CAD build for the part. Positions are in the model's coordinates, mm. A direction names the side the tool comes from. Coordinates: 2 decimals unless noted, no trailing zeros. Order: outer loops, then holes, each group sorted by start corner. A loop starts at its lowest first (then second) coordinate and runs counter-clockwise, first axis right, second up. Notation, with made-up numbers: M -11.5,32.25 L 25.5,32.25 A16 ccw 25.5,44.25 Z; hole C 26,76.25 d3. An arc over 180 degrees is marked long. One line per item, written item: value.
from build123d import *

# Parameters (mm, degrees)
SKETCH1_W           = 244
SKETCH1_H           = 158.154567899
BOSS_EXTRUDE2_DEPTH = 5
SKETCH2_W           = 28.286613298
SKETCH2_H           = 62.131328865
CUT_EXTRUDE1_DEPTH  = 10
SKETCH7_W           = 32
SKETCH7_H           = 84.5
CUT_EXTRUDE5_DEPTH  = 10
SKETCH9_R           = 1.5
CUT_EXTRUDE7_DEPTH  = 10
SKETCH10_W          = 26
SKETCH10_H          = 40
CUT_EXTRUDE8_DEPTH  = 10
SKETCH12_W          = 92
SKETCH12_H          = 45
CUT_EXTRUDE10_DEPTH = 10
SKETCH13_R          = 2.5
CUT_EXTRUDE11_DEPTH = 10
CUT_EXTRUDE12_DEPTH = 10
SKETCH15_W          = 32
SKETCH15_H          = 26
BOSS_EXTRUDE3_DEPTH = 5
SKETCH16_R          = 1.5
CUT_EXTRUDE13_DEPTH = 10
SKETCH17_R          = 1.5
CUT_EXTRUDE14_DEPTH = 10
SKETCH19_R          = 2
CUT_EXTRUDE16_DEPTH = 10
SKETCH20_W          = 22
SKETCH20_H          = 28
CUT_EXTRUDE17_DEPTH = 10
CUT_EXTRUDE18_DEPTH = 10


with BuildPart() as part:
    # Sketch1 → Boss-Extrude2 (new body)
    with BuildSketch(Plane.XY):
        with Locations((-3, -45.239754423)):
            Rectangle(SKETCH1_W, SKETCH1_H)
    extrude(amount=BOSS_EXTRUDE2_DEPTH)

    # Sketch2 → Cut-Extrude1 (cut)
    with BuildSketch(Plane(origin=(0, 0, 0), x_dir=(-1, 0, 0), z_dir=(0, 0, -1))):
        with Locations((50, -93.25137394)):
            Rectangle(SKETCH2_W, SKETCH2_H)
    extrude(amount=-CUT_EXTRUDE1_DEPTH, mode=Mode.SUBTRACT)

    # Sketch7 → Cut-Extrude5 (cut)
    with BuildSketch(Plane(origin=(0, 0, 0), x_dir=(-1, 0, 0), z_dir=(0, 0, -1))):
        with Locations((-103, -40.912470473)):
            Rectangle(SKETCH7_W, SKETCH7_H)
    extrude(amount=-CUT_EXTRUDE5_DEPTH, mode=Mode.SUBTRACT)

    # Sketch9 → Cut-Extrude7 (cut)
    with BuildSketch(Plane(origin=(0, 0, 0), x_dir=(-1, 0, 0), z_dir=(0, 0, -1))):
        with Locations((31.026566737, -67.835709507)):
            Circle(SKETCH9_R)
        with Locations((31.026566737, -82.835709507)):
            Circle(SKETCH9_R)
    extrude(amount=-CUT_EXTRUDE7_DEPTH, mode=Mode.SUBTRACT)

    # Sketch10 → Cut-Extrude8 (cut)
    with BuildSketch(Plane(origin=(0, 0, 0), x_dir=(-1, 0, 0), z_dir=(0, 0, -1))):
        with Locations((3, -104.317038372)):
            Rectangle(SKETCH10_W, SKETCH10_H)
    extrude(amount=-CUT_EXTRUDE8_DEPTH, mode=Mode.SUBTRACT)

    # Sketch12 → Cut-Extrude10 (cut)
    with BuildSketch(Plane(origin=(0, 0, 0), x_dir=(-1, 0, 0), z_dir=(0, 0, -1))):
        with Locations((-3, 11.337529527)):
            Rectangle(SKETCH12_W, SKETCH12_H)
    extrude(amount=-CUT_EXTRUDE10_DEPTH, mode=Mode.SUBTRACT)

    # Sketch13 → Cut-Extrude11 (cut)
    with BuildSketch(Plane(origin=(0, 0, 0), x_dir=(-1, 0, 0), z_dir=(0, 0, -1))):
        with Locations((-107, -109.317038372)):
            Circle(SKETCH13_R)
        with Locations((113, -109.317038372)):
            Circle(SKETCH13_R)
        with Locations((-62, 13.837529527)):
            Circle(SKETCH13_R)
        with Locations((68, 13.837529527)):
            Circle(SKETCH13_R)
    extrude(amount=-CUT_EXTRUDE11_DEPTH, mode=Mode.SUBTRACT)

    # Sketch14 → Cut-Extrude12 (cut)
    with BuildSketch(Plane(origin=(0, 0, 0), x_dir=(-1, 0, 0), z_dir=(0, 0, -1))):
        Polygon((-119, -94.885674772), (-119, -98.885674772), (-111.613125162, -98.885674772), (-111.613125162, -99.635674772), (-109.213125162, -99.635674772), (-109.213125162, -98.885674772), (-102, -98.885674772), (-102, -94.885674772), (-109.213125162, -94.885674772), (-109.213125162, -94.135674772), (-111.613125162, -94.135674772), (-111.613125162, -94.885674772), align=None)
        Polygon((-102, 11.114325228), (-109.213125162, 11.114325228), (-109.213125162, 11.864325228), (-111.613125162, 11.864325228), (-111.613125162, 11.114325228), (-119, 11.114325228), (-119, 7.114325228), (-111.613125162, 7.114325228), (-111.613125162, 6.364325228), (-109.213125162, 6.364325228), (-109.213125162, 7.114325228), (-102, 7.114325228), align=None)
        Polygon((117.613125162, 7.114325228), (125, 7.114325228), (125, 11.114325228), (117.613125162, 11.114325228), (117.613125162, 11.864325228), (115.213125162, 11.864325228), (115.213125162, 11.114325228), (108, 11.114325228), (108, 7.114325228), (115.213125162, 7.114325228), (115.213125162, 6.364325228), (117.613125162, 6.364325228), align=None)
        Polygon((117.613125162, -98.885674772), (125, -98.885674772), (125, -94.885674772), (117.613125162, -94.885674772), (117.613125162, -94.135674772), (115.213125162, -94.135674772), (115.213125162, -94.885674772), (108, -94.885674772), (108, -98.885674772), (115.213125162, -98.885674772), (115.213125162, -99.635674772), (117.613125162, -99.635674772), align=None)
    extrude(amount=-CUT_EXTRUDE12_DEPTH, mode=Mode.SUBTRACT)

    # Sketch15 → Boss-Extrude3 (add)
    with BuildSketch(Plane(origin=(0, 0, 0), x_dir=(-1, 0, 0), z_dir=(0, 0, -1))):
        with Locations((-103, -11.662470473)):
            Rectangle(SKETCH15_W, SKETCH15_H)
    extrude(amount=-BOSS_EXTRUDE3_DEPTH)

    # Sketch16 → Cut-Extrude13 (cut)
    with BuildSketch(Plane(origin=(0, 0, 0), x_dir=(-1, 0, 0), z_dir=(0, 0, -1))):
        with Locations((-69.5, -5.762708109)):
            Circle(SKETCH16_R)
        with Locations((-69.5, -15.762708109)):
            Circle(SKETCH16_R)
    extrude(amount=-CUT_EXTRUDE13_DEPTH, mode=Mode.SUBTRACT)

    # Sketch17 → Cut-Extrude14 (cut)
    with BuildSketch(Plane(origin=(0, 0, 0), x_dir=(-1, 0, 0), z_dir=(0, 0, -1))):
        with Locations((-69, 16.337529527)):
            Circle(SKETCH17_R)
        with Locations((-69, 29.337529527)):
            Circle(SKETCH17_R)
        with Locations((-116, 16.337529527)):
            Circle(SKETCH17_R)
        with Locations((-116, 29.337529527)):
            Circle(SKETCH17_R)
    extrude(amount=-CUT_EXTRUDE14_DEPTH, mode=Mode.SUBTRACT)

    # Sketch19 → Cut-Extrude16 (cut)
    with BuildSketch(Plane(origin=(0, 0, 0), x_dir=(-1, 0, 0), z_dir=(0, 0, -1))):
        with Locations((33, -34.730312102)):
            Circle(SKETCH19_R)
        with Locations((47, -34.730312102)):
            Circle(SKETCH19_R)
        with Locations((33, -50.230312102)):
            Circle(SKETCH19_R)
        with Locations((47, -50.230312102)):
            Circle(SKETCH19_R)
    extrude(amount=-CUT_EXTRUDE16_DEPTH, mode=Mode.SUBTRACT)

    # Sketch20 → Cut-Extrude17 (cut)
    with BuildSketch(Plane(origin=(0, 0, 0), x_dir=(-1, 0, 0), z_dir=(0, 0, -1))):
        with Locations((-65.5, -110.317038372)):
            Rectangle(SKETCH20_W, SKETCH20_H)
    extrude(amount=-CUT_EXTRUDE17_DEPTH, mode=Mode.SUBTRACT)

    # Sketch21 → Cut-Extrude18 (cut)
    with BuildSketch(Plane(origin=(0, 0, 0), x_dir=(-1, 0, 0), z_dir=(0, 0, -1))):
        with BuildLine():
            Line((-29, -36.162470473), (-69, -36.162470473))
            ThreePointArc((-69, -36.162470473), (-74.402823378, -41.565293851), (-69, -46.968117229))
            Line((-69, -46.968117229), (-29, -46.968117229))
            ThreePointArc((-29, -46.968117229), (-23.597176622, -41.565293851), (-29, -36.162470473))
        make_face()
        with BuildLine():
            Line((115, -36.162470473), (75, -36.162470473))
            ThreePointArc((75, -36.162470473), (69.597176622, -41.565293851), (75, -46.968117229))
            Line((75, -46.968117229), (115, -46.968117229))
            ThreePointArc((115, -46.968117229), (120.402823378, -41.565293851), (115, -36.162470473))
        make_face()
    extrude(amount=-CUT_EXTRUDE18_DEPTH, mode=Mode.SUBTRACT)


solid = part.part
Q1. Mould opens along Y. For faces 1 (the face through (-115.3, -110.3, 2.5)), 2 (the face through (84, 33.838, 2)), 3 (the face through (10, -105, 2)) say: released by +Y, released by -Y, zero draft, split by the parting line, or undercut.
Recorded:
face 1: undercut
face 2: released by +Y
face 3: zero draft
Q2. Drill centre lines: line 1 along X through (y, z) = (-100, 4.1); line 2 along Y through (x, z) = (116, 1.55); line 3 along X through (y, z) = (-94, 0.5). Where is each one in solid material? Low to high.
Recorded:
line 1: x = -125 to -64.14, -35.86 to -16, 10 to 54.5, 76.5 to 119
line 2: y = -124.32 to -98.89, -94.89 to -83.16, -24.66 to 7.11, 11.11 to 14.84, 17.84 to 27.84, 30.84 to 33.84
line 3: x = -125 to -64.14, -35.86 to -16, 10 to 119
Q3. Slice it at A-A (y = -90). List the corners of the cut face in (x, z), plus the area to 3 significant figures.
Recorded:
outline: M -125,0 L -64.14,0 L -64.14,5 L -125,5 Z; M -35.86,0 L -16,0 L -16,5 L -35.86,5 Z; M 10,0 L 119,0 L 119,5 L 10,5 Z
area: 949 mm^2
Q4. Which spindle directions (+Z, -Z, +X, -X, +Y, -Y) get a long thin tool onto all of the face, cutting with end or side? Do faces 4 (the face through (103, -24.662, 2)), 5 (the face through (4, -11.162, 2)), 6 (the face through (-121, -94.886, 2)), 7 (the face through (49, -36.162, 2)). Say none if no direction does.
Recorded:
face 4: +Z, -Z, +X
face 5: +Z, -Z, +Y
face 6: +Z, -Z, -X
face 7: +Z, -Z
Q5. Slice it at C-C (y = -73). List the corners of the cut face in (x, z), plus the area to 3 significant figures.
Recorded:
outline: M -125,0 L -64.14,0 L -64.14,5 L -125,5 Z; M -35.86,0 L 87,0 L 87,5 L -35.86,5 Z
area: 919 mm^2
Q6. Pin check, flat tips, straight feed: pin 1 Ø1.5 at (x, z) = (66.5, 3.5) entering from -Y; pin 2 Ø1.5 at (x, z) = (2, 3) entering from -Y; pin 3 Ø1.5 at (x, z) = (45.5, 3) entering from +Y; pin 4 Ø6 at (x, y) = (27.5, -19.5) entering from -Z. Stop position of each tip, or through.
Recorded:
pin 1: stops at y = -96.32
pin 2: stops at y = -84.32
pin 3: stops at y = -11.16
pin 4: stops at z = 0
Q7. Slice it at B-B (x = 62). List the corners of the cut face in (y, z), plus the area to 3 significant figures.
Recorded:
outline: M -96.32,0 L -46.97,0 L -46.97,5 L -96.32,5 Z; M -36.16,0 L 11.34,0 L 11.34,5 L -36.16,5 Z; M 16.34,0 L 33.84,0 L 33.84,5 L 16.34,5 Z
area: 572 mm^2
Q8. Slice it at D-D (x = 91.5). List the corners of the cut face in (y, z), plus the area to 3 significant figures.
Recorded:
outline: M -124.32,0 L -83.16,0 L -83.16,5 L -124.32,5 Z; M -24.66,0 L 33.84,0 L 33.84,5 L -24.66,5 Z
area: 498 mm^2
